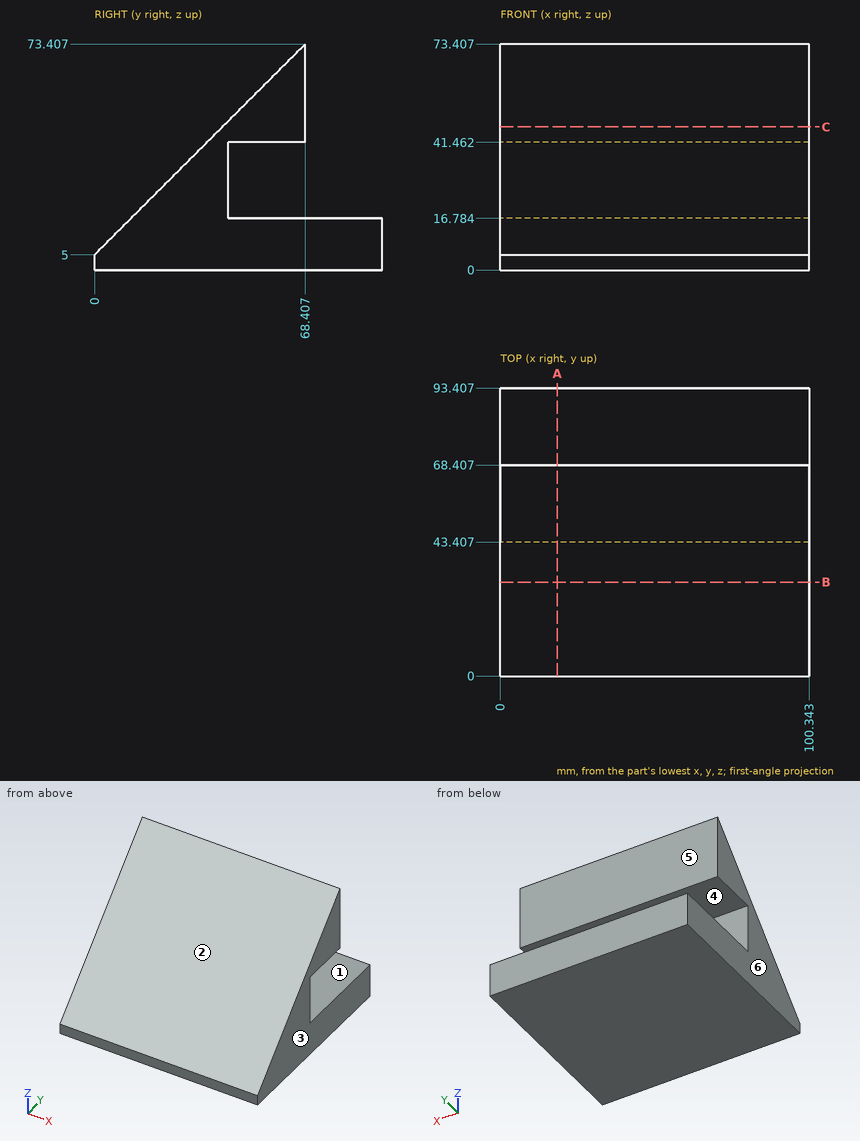
Geometry: see drawing. Coordinates: mm, zero at the bounding-box minimum. A direction names the side the tool comes from. Round coordinates to 2 decimals unless told otherwise and drop trailing zeros. Order: outer loops, then holes, each group sorted by start corner. A loop starts at its lowest first (then second) coordinate and runs counter-clockwise, first axis right, second up. Notation, with made-up numbers: (9.25, -8) - (51.25, -8) arc R12 cw to (51.25, -1) - close; hole circle Ø9 at (18.25, 31). An arc over 180 degrees is marked (long way). Use a Markdown table: item, result. Add a question column.
1. Line query: probe 1 along Z at (x, y) = (28.5, 88); probe 2 along Z at (x, y) = (55, 51) (1 decimal); probe 3 along Z at (x, y) = (18.5, 65) (1 decimal). Output: solid intervals per line, ascending.
2. Section query B-B (y = 30.5). Return the cut outline in (x, z), then the cut area to 3 significant figures.
3. Mould query, pull axis Z, two halves, no side actions, for the marked faces 1, 2 and 3. Classes: +Z half, -Z half, draft (parallel to the pull), parting line (faces both ways), or undercut.
4. Set-up query: the marked faces 4, 5 and 6. Return all of +Z, -Z, +X, -X, +Y, -Y with unobstructed straight access to the full face (end or side cutting, diameter ignored); none if empty.
5. Section query A-A (x = 18.5). Return the cut outline in (y, z), then the cut area to 3 significant figures.
6. Section query C-C (z = 46.5). Return the cut outline in (x, y), then the cut area to 3 significant figures.
7. First-contact query: pin 1 (20 mm diameter, centred on x = 55, y = 55, fed in from -Z); pin 2 (5 mm diameter, centred on x = 18.5, z = 13.5, fed in from -Y); pin 3 (8 mm diameter, centred on x = 14, z = 62, fed in from -Y); pin 4 (7.5 mm diameter, centred on x = 38, z = 29, fed in from +Y). Flat tips, straight axial feed; report the tip coordinate or a pass-through.
Derived:
| question | item | result |
|---|---|---|
| 1 | probe 1 | 0 to 16.78 |
| 1 | probe 2 | 0 to 16.8, 41.5 to 56 |
| 1 | probe 3 | 0 to 16.8, 41.5 to 70 |
| 2 | outline | (0, 0) - (100.34, 0) - (100.34, 35.5) - (0, 35.5) - close |
| 2 | area | 3,560 mm2 |
| 3 | face 1 | undercut |
| 3 | face 2 | +Z half |
| 3 | face 3 | draft |
| 4 | face 4 | +X, -X, +Y |
| 4 | face 5 | +Z, +X, -X, +Y |
| 4 | face 6 | +Z, -Z, -X, +Y, -Y |
| 5 | outline | (0, 0) - (93.41, 0) - (93.41, 16.78) - (43.41, 16.78) - (43.41, 41.46) - (68.41, 41.46) - (68.41, 73.41) - (0, 5) - close |
| 5 | area | 2,480 mm2 |
| 6 | outline | (0, 41.5) - (100.34, 41.5) - (100.34, 68.41) - (0, 68.41) - close |
| 6 | area | 2,700 mm2 |
| 7 | pin 1 | z = 0 |
| 7 | pin 2 | y = 6 |
| 7 | pin 3 | y = 53 |
| 7 | pin 4 | y = 43.41 |
